```python
from build123d import *

# Parameters (mm, degrees)
BOSS_EXTRUDE1_DEPTH            = 81.28
SKETCH3_W                      = 76.2
SKETCH3_H                      = 50.292
CUT_EXTRUDE1_DEPTH             = 37.846
SKETCH4_W                      = 40.386
SKETCH4_H                      = 43.18
CUT_EXTRUDE2_DEPTH             = 52.832
FILLET1_R                      = 2.54
FILLET2_R                      = 2.54
FILLET3_R                      = 2.54
FILLET4_R                      = 2.54
SKETCH7_W                      = 16.51
SKETCH7_H                      = 2.54
CUT_EXTRUDE4_REACH             = 54.566
SKETCH8_W                      = 16.51
SKETCH8_H                      = 16.012242806
CUT_EXTRUDE4_DIRECTION_2_DEPTH = 2.54
FILLET5_R                      = 1.27


with BuildPart() as part:
    # Sketch1 → Boss-Extrude1 (new body)
    with BuildSketch(Plane.XY):
        with BuildLine():
            Line((0, 52.9844), (0, 58.0644))
            ThreePointArc((0, 58.0644), (12.7, 70.7644), (0, 83.4644))
            Line((0, 83.4644), (0, 98.7044))
            Line((0, 98.7044), (40.386, 98.7044))
            Line((40.386, 98.7044), (40.386, 25.398729968))
            ThreePointArc((40.386, 25.398729968), (40.827682914, 17.344312358), (42.147434783, 9.386487162))
            ThreePointArc((42.147434783, 9.386487162), (33.688432107, -27.011144777), (0, -43.18))
            Line((0, -43.18), (0, -35.2044))
            ThreePointArc((0, -35.2044), (35.2044, 0), (0, 35.2044))
            Line((0, 35.2044), (0, 52.9844))
        make_face()
    extrude(amount=-BOSS_EXTRUDE1_DEPTH)

    # Sketch3 → Cut-Extrude1 (cut)
    with BuildSketch(Plane.ZY):
        with Locations((-40.64, 71.0184)):
            Rectangle(SKETCH3_W, SKETCH3_H)
    extrude(amount=-CUT_EXTRUDE1_DEPTH, mode=Mode.SUBTRACT)

    # Sketch4 → Cut-Extrude2 (cut)
    with BuildSketch(Plane(origin=(0, 98.7044, 0), x_dir=(1, 0, 0), z_dir=(0, 1, 0))):
        with Locations((20.193, 40.64)):
            Rectangle(SKETCH4_W, SKETCH4_H)
    extrude(amount=-CUT_EXTRUDE2_DEPTH, mode=Mode.SUBTRACT)

    # Fillet1
    fillet1_edges = [part.edges().sort_by_distance(p)[0] for p in [
        (18.923, 45.8724, -78.74),
        (18.923, 45.8724, -2.54),
        (37.846, 45.8724, -10.795),
        (37.846, 45.8724, -70.485),
    ]]
    fillet(fillet1_edges, radius=FILLET1_R)

    # Fillet2
    fillet2_edges = [part.edges().sort_by_distance(p)[0] for p in [
        (37.846, 96.1644, -70.485),
        (37.846, 96.1644, -10.795),
    ]]
    fillet(fillet2_edges, radius=FILLET2_R)

    # Fillet3
    fillet3_edges = [part.edges().sort_by_distance(p)[0] for p in [
        (36.576, 45.8724, -19.05),
        (36.576, 45.8724, -62.23),
    ]]
    fillet(fillet3_edges, radius=FILLET3_R)

    # Fillet4
    fillet4_edges = [part.edges().sort_by_distance(p)[0] for p in [
        (40.386, 98.7044, -71.755),
        (40.386, 98.7044, -9.525),
    ]]
    fillet(fillet4_edges, radius=FILLET4_R)

    # Sketch7 → Cut-Revolve2 (revolve, cut)
    with BuildSketch(Plane.ZY):
        with Locations((-40.64, -41.91)):
            Rectangle(SKETCH7_W, SKETCH7_H)
    revolve(axis=Axis((0, 0, -81.28), (0, 0, 1)), mode=Mode.SUBTRACT)

    # Sketch8 → Cut-Extrude4 (cut, up to next)
    with BuildSketch(Plane(origin=(42.147434783, 9.386487162, 0), x_dir=(0, 0, -1), z_dir=(0.976086957, 0.217380435, 0)), mode=Mode.PRIVATE) as cut_extrude4_sk1:
        with Locations((40.64, 8.006121403)):
            Rectangle(SKETCH8_W, SKETCH8_H)
    cut_extrude4_tool1 = extrude(cut_extrude4_sk1.sketch, amount=-CUT_EXTRUDE4_REACH, mode=Mode.PRIVATE) & part.part
    add(cut_extrude4_tool1.solids().sort_by_distance((40.407061, 17.201158, -40.64))[0], mode=Mode.SUBTRACT)

    # Sketch8 → Cut-Extrude4 direction 2 (cut)
    with BuildSketch(Plane(origin=(42.147434783, 9.386487162, 0), x_dir=(0, 0, -1), z_dir=(0.976086957, 0.217380435, 0))):
        with Locations((40.64, 8.006121403)):
            Rectangle(SKETCH8_W, SKETCH8_H)
    extrude(amount=CUT_EXTRUDE4_DIRECTION_2_DEPTH, mode=Mode.SUBTRACT)

    # Fillet5
    fillet5_edges = [part.edges().sort_by_distance(p)[0] for p in [
        (40.64, 0, -48.895),
        (40.64, 0, -32.385),
    ]]
    fillet(fillet5_edges, radius=FILLET5_R)


solid = part.part
```
Input: part model. Units: mm. Frame: model coordinates. A direction names the side the tool comes from. Round coordinates to 2 decimals unless told otherwise and drop trailing zeros. Loops run counter-clockwise (first coordinate to the right, second up) from the corner with the lowest first, then second, coordinate; pieces in that order, holes last.
1) Pin query (flat end, axial travel): pin 1 (1.5 mm diameter, centred on x = 27, z = -51.5, fed in from -Y); pin 2 (5 mm diameter, centred on y = 76.5, z = -73.5, fed in from -X); pin 3 (8.5 mm diameter, centred on x = 23, z = -67, fed in from -Y). Return the tip coordinate at first contact, or that it passes through.
Ans:
pin 1: stops at y = -34.28
pin 2: stops at x = 37.85
pin 3: stops at y = -38.9
2) Material intervals for line 1 (Z direction, x = 27, y = 56.5); line 2 (Y direction, x = 26.5, z = -64); line 3 (Z direction, x = 38, y = -17.5), sorted ascending.
Ans:
line 1: z = -81.28 to -78.74, -2.54 to 0
line 2: y = -34.09 to -23.18, 23.18 to 45.87, 96.16 to 98.7
line 3: z = -81.28 to -48.89, -32.39 to 0
3) Section query C-C on x = 27. Count the separate pieces of the cut face and the enclosed holes in it, plus the area to 3 significant figures.
Ans:
separate pieces: 2
enclosed holes: 1
area: 3,040 mm2
4) Section query A-A on y = 61.5. Return the cut outline in (x, z).
Ans:
outline: (8.69, -81.28) - (40.39, -81.28) - (40.39, -62.23) - (37.85, -62.23) - (37.85, -78.74) - (8.69, -78.74) - close; (8.69, -2.54) - (37.85, -2.54) - (37.85, -19.05) - (40.39, -19.05) - (40.39, 0) - (8.69, 0) - close
5) Section query D-D on y = 0. Return the cut outline in (x, z) (3 decimals).
Ans:
outline: (35.204, -81.28) - (43.18, -81.28) - (43.18, -48.895) - (41.91, -48.895) arc R1.27 cw to (40.64, -47.625) - (40.64, -33.655) arc R1.27 cw to (41.91, -32.385) - (43.18, -32.385) - (43.18, 0) - (35.204, 0) - close
6) Set-up query: faces 4 (the flat face through (0, 39, -40)), 5 (the cylindrical face through (37.082, 46.597, -11.932)), 6 (the flat face through (38, 81, -19.05)), 7 (the flat face through (37.991, 24.865, -40.524)). Return all of +Z, -Z, +X, -X, +Y, -Y with unobstructed straight access to the full face (end or side cutting, diameter ignored); none if empty.
Ans:
face 4: +Z, -Z, -X, +Y, -Y
face 5: -X
face 6: +X, -X, +Y
face 7: +X
7) Pull-direction query (Y, two-part tool) for faces 1 (the flat face through (0, -39, -40)), 2 (the flat face through (19, 98.704, -9)), 3 (the flat face through (20, 45.872, -41)); classes: released by +Y, released by -Y, zero draft, split by the parting line, or undercut.
Ans:
face 1: zero draft
face 2: released by +Y
face 3: undercut
8) Section query B-B on z = -10. Return the cut outline in (x, y).
Ans:
outline: (0, -43.18) arc R43.18 ccw to (42.15, 9.39) arc R73.66 cw to (40.39, 25.4) - (40.39, 96.16) arc R2.54 ccw to (37.85, 98.7) - (0, 98.7) - (0, 96.16) - (35.31, 96.16) arc R2.54 cw to (37.85, 93.62) - (37.85, 48.41) arc R2.54 cw to (35.31, 45.87) - (0, 45.87) - (0, 35.2) arc R35.2 cw to (0, -35.2) - close
